Could you check a few things on this model? Use its own coordinates, in mm. A direction names the side the tool comes from. Round coordinates to 2 decimals unless told otherwise and drop trailing zeros. Loops run counter-clockwise (first coordinate to the right, second up) from the corner with the lowest first, then second, coordinate; pieces in that order, holes last. Notation, with made-up numbers: (51, 62) -> (93, 62) arc R26 cw to (93, 78) -> close; hole circle Ø5 at (12.5, 1.5). An arc over 180 degrees is marked (long way). Put each result on its own line as item: value. Start each with the question number.
1. I'm going to push flat-ended pins straight in: P1, Ø3, axis at y = -2, z = 98.5, coming from the +X side; P2, Ø8, axis at x = 10, y = 2.5, coming from the +Z side. Where does each tip first touch, or does it pass through?
2. I need wall thicknesses on line 1 (Y direction, x = 7.5, z = 85.5); line 2 (Y direction, x = 4, z = 42.5) (3 decimals); line 3 (X direction, y = -0.75, z = 197). Which ranges of each line are inside material? Lowest first, please. Write a range as [from, to].
3. Imagine slicing it at B-B, the plane x = 0.25. Please give me the cut outline in (y, z) (3 decimals), and give its area (3 significant figures).
4. Imagine slicing it at A-A, the plane y = 0. Please give me the cut outline in (x, z), and give its area (3 significant figures).
5. Which directions (+Z, -Z, +X, -X, +Y, -Y) give clear straight access to the entire face, cutting with the end or side of a thin tool? Please do faces 1 (the flat face through (0, -6.025, 135)), 2 (the flat face through (0.1, -6.3, 0)).
6. If we mould it in two halves opening along Y, with no side actions, what happens to faces 3 (the flat face through (0.1, -6.3, 273.05)), 4 (the flat face through (0, 6.025, 135)), 5 (the cylindrical face through (14.5, 0.17, 134.61))? For each: pulls with the +Y half, pulls with the -Y half, needs draft (parallel to the pull), parting line crosses it, or undercut.
7. Imagine slicing it at C-C, the plane z = 101.5. Please give me the cut outline in (x, y) (3 decimals).
```python
from build123d import *

# Parameters (mm, degrees)
BOSS_EXTRUDE1_DEPTH     = 273.05
CUT_EXTRUDE1_DEPTH      = 274.544539335
CUT_EXTRUDE1_DEPTH_BACK = 274.544539335


with BuildPart() as part:
    # Sketch1 → Boss-Extrude1 (new body)
    with BuildSketch(Plane.XY):
        with BuildLine():
            Line((-6.75, 7.75), (6.75, 7.75))
            ThreePointArc((6.75, 7.75), (14.5, 0), (6.75, -7.75))
            Line((6.75, -7.75), (-6.75, -7.75))
            ThreePointArc((-6.75, -7.75), (-14.5, 0), (-6.75, 7.75))
        make_face()
    extrude(amount=BOSS_EXTRUDE1_DEPTH)

    # Sketch2 → Cut-Extrude1 (cut, two sides: drawn at the far end of the back side and taken through both)
    with BuildSketch(Plane.XY.offset(273.05).offset(-CUT_EXTRUDE1_DEPTH_BACK)):
        with BuildLine():
            Line((-7.475, 6.025), (7.475, 6.025))
            ThreePointArc((7.475, 6.025), (13.5, 0), (7.475, -6.025))
            Line((7.475, -6.025), (-7.475, -6.025))
            ThreePointArc((-7.475, -6.025), (-13.5, 0), (-7.475, 6.025))
        make_face()
    extrude(amount=CUT_EXTRUDE1_DEPTH + CUT_EXTRUDE1_DEPTH_BACK, mode=Mode.SUBTRACT)


solid = part.part
```
Entries:
1. P1: x = 14.48
1. P2: z = 273.05
2. line 1: [-7.71, -6.02], [6.02, 7.71]
2. line 2: [-7.75, -6.025], [6.025, 7.75]
2. line 3: [-14.46, -13.45], [13.45, 14.46]
3. outline: (-7.75, 0) -> (-6.025, 0) -> (-6.025, 273.05) -> (-7.75, 273.05) -> close; (6.025, 0) -> (7.75, 0) -> (7.75, 273.05) -> (6.025, 273.05) -> close
3. area: 942 mm^2
4. outline: (-14.5, 0) -> (-13.5, 0) -> (-13.5, 273.05) -> (-14.5, 273.05) -> close; (13.5, 0) -> (14.5, 0) -> (14.5, 273.05) -> (13.5, 273.05) -> close
4. area: 546 mm^2
5. face 1: +Z, -Z
5. face 2: -Z, +X, -X, +Y, -Y
6. face 3: needs draft
6. face 4: undercut
6. face 5: parting line crosses it
7. outline: (-6.75, -7.75) -> (6.75, -7.75) arc R7.75 ccw to (6.75, 7.75) -> (-6.75, 7.75) arc R7.75 ccw to start; hole (-7.475, -6.025) -> (7.475, -6.025) arc R6.025 ccw to (7.475, 6.025) -> (-7.475, 6.025) arc R6.025 ccw to start
